Input: part model. Units: mm. Frame: model coordinates. Round coordinates to 2 decimals unless told otherwise and drop trailing zeros. Write each loop counter-clockwise with the first axis right and the second up, starting at its lowest first coordinate (ties: lowest second). Pieces come first, ordered by that corner, then holes. Notation, with made-up numbers: (16.5, -14) -> (67.5, -14) arc R10 cw to (67.5, -9) -> close; hole circle Ø9 at (27, 27). An arc over 180 degrees is marked (long way). Write item = value, one per line. Start each with the question number.
```python
from build123d import *

# Parameters (mm, degrees)
SKETCH1_R           = 2.265
BOSS_EXTRUDE1_DEPTH = 3
SKETCH2_W           = 6.5
SKETCH2_H           = 20
CUT_EXTRUDE1_DEPTH  = 3
BOSS_EXTRUDE2_DEPTH = 3
CUT_EXTRUDE2_DEPTH  = 3
SKETCH5_W           = 3
SKETCH5_H           = 20
BOSS_EXTRUDE3_DEPTH = 3
SKETCH6_W           = 27.010134686
SKETCH6_H           = 17.9
CUT_EXTRUDE3_DEPTH  = 3
SKETCH7_W           = 19.5
SKETCH7_H           = 14.6
CUT_EXTRUDE4_DEPTH  = 3
SKETCH8_W           = 19.5
SKETCH8_H           = 15.6
CUT_EXTRUDE5_DEPTH  = 3
SKETCH9_W           = 2.019620965
SKETCH9_H           = 0.574286347
CUT_EXTRUDE6_DEPTH  = 3
SKETCH10_W          = 15
SKETCH10_H          = 3
CUT_EXTRUDE7_DEPTH  = 3
FILLET1_R           = 0.6


with BuildPart() as part:
    # Sketch1 → Boss-Extrude1 (new body)
    with BuildSketch(Plane(origin=(0, 0, 0), x_dir=(1, 0, 0), z_dir=(0, 1, 0))):
        with BuildLine():
            Line((4.265, 0), (87.735, 0))
            ThreePointArc((87.735, 0), (95.015810422, 3.015810422), (92, -4.265))
            Line((92, -4.265), (92, -58.735))
            ThreePointArc((92, -58.735), (95.015810422, -66.015810422), (87.735, -63))
            Line((87.735, -63), (4.265, -63))
            ThreePointArc((4.265, -63), (-3.015810422, -66.015810422), (0, -58.735))
            Line((0, -58.735), (0, -4.265))
            ThreePointArc((0, -4.265), (-3.015810422, 3.015810422), (4.265, 0))
        make_face()
        with Locations(Location((0, 0, 0), (0, 0, 270))):
            Circle(SKETCH1_R, mode=Mode.SUBTRACT)
        with Locations(Location((92, 0, 0), (0, 0, 270))):
            Circle(SKETCH1_R, mode=Mode.SUBTRACT)
        with Locations(Location((92, -63, 0), (0, 0, 270))):
            Circle(SKETCH1_R, mode=Mode.SUBTRACT)
        with Locations(Location((0, -63, 0), (0, 0, 270))):
            Circle(SKETCH1_R, mode=Mode.SUBTRACT)
    extrude(amount=BOSS_EXTRUDE1_DEPTH)

    # Sketch2 → Cut-Extrude1 (cut)
    with BuildSketch(Plane(origin=(0, 3, 0), x_dir=(1, 0, 0), z_dir=(0, 1, 0))):
        with Locations((3.25, -31.5)):
            Rectangle(SKETCH2_W, SKETCH2_H)
    extrude(amount=-CUT_EXTRUDE1_DEPTH, mode=Mode.SUBTRACT)

    # Sketch3 → Boss-Extrude2 (add)
    with BuildSketch(Plane(origin=(0, 3, 0), x_dir=(1, 0, 0), z_dir=(0, 1, 0))):
        with BuildLine():
            Line((-2.7, -15.5), (0, -14.9))
            Line((0, -14.9), (0, -21.5))
            Line((0, -21.5), (-2.5, -21.5))
            ThreePointArc((-2.5, -21.5), (-2.853553391, -21.353553391), (-3, -21))
            Line((-3, -21), (-3, -15.8))
            ThreePointArc((-3, -15.8), (-2.912132034, -15.587867966), (-2.7, -15.5))
        make_face()
        with BuildLine():
            Line((-3, -42), (-3, -47.2))
            ThreePointArc((-3, -47.2), (-2.912132034, -47.412132034), (-2.7, -47.5))
            Line((-2.7, -47.5), (0, -48.1))
            Line((0, -48.1), (0, -41.5))
            Line((0, -41.5), (-2.5, -41.5))
            ThreePointArc((-2.5, -41.5), (-2.853553391, -41.646446609), (-3, -42))
        make_face()
    extrude(amount=-BOSS_EXTRUDE2_DEPTH)

    # Sketch4 → Cut-Extrude2 (cut)
    with BuildSketch(Plane(origin=(0, 3, 0), x_dir=(1, 0, 0), z_dir=(0, 1, 0))):
        with BuildLine():
            Line((6, -3), (64, -3))
            ThreePointArc((64, -3), (66.121320344, -3.878679656), (67, -6))
            Line((67, -6), (67, -57))
            ThreePointArc((67, -57), (66.121320344, -59.121320344), (64, -60))
            Line((64, -60), (6, -60))
            ThreePointArc((6, -60), (3.878679656, -59.121320344), (3, -57))
            Line((3, -57), (3, -6))
            ThreePointArc((3, -6), (3.878679656, -3.878679656), (6, -3))
        make_face()
    extrude(amount=-CUT_EXTRUDE2_DEPTH, mode=Mode.SUBTRACT)

    # Sketch5 → Boss-Extrude3 (add)
    with BuildSketch(Plane(origin=(0, 3, 0), x_dir=(1, 0, 0), z_dir=(0, 1, 0))):
        with Locations((1.5, -31.5)):
            Rectangle(SKETCH5_W, SKETCH5_H)
    extrude(amount=-BOSS_EXTRUDE3_DEPTH)

    # Sketch6 → Cut-Extrude3 (cut)
    with BuildSketch(Plane(origin=(0, 3, 0), x_dir=(1, 0, 0), z_dir=(0, 1, 0))):
        with Locations((82.505067343, -14.45)):
            Rectangle(SKETCH6_W, SKETCH6_H)
    extrude(amount=-CUT_EXTRUDE3_DEPTH, mode=Mode.SUBTRACT)

    # Sketch7 → Cut-Extrude4 (cut)
    with BuildSketch(Plane(origin=(0, 3, 0), x_dir=(1, 0, 0), z_dir=(0, 1, 0))):
        with Locations((82.25, -33.7)):
            Rectangle(SKETCH7_W, SKETCH7_H)
    extrude(amount=-CUT_EXTRUDE4_DEPTH, mode=Mode.SUBTRACT)

    # Sketch8 → Cut-Extrude5 (cut)
    with BuildSketch(Plane(origin=(0, 3, 0), x_dir=(1, 0, 0), z_dir=(0, 1, 0))):
        with Locations((82.25, -51.3)):
            Rectangle(SKETCH8_W, SKETCH8_H)
    extrude(amount=-CUT_EXTRUDE5_DEPTH, mode=Mode.SUBTRACT)

    # Sketch9 → Cut-Extrude6 (cut)
    with BuildSketch(Plane(origin=(0, 3, 0), x_dir=(1, 0, 0), z_dir=(0, 1, 0))):
        with Locations((93.009810483, -58.812856827)):
            Rectangle(SKETCH9_W, SKETCH9_H)
    extrude(amount=-CUT_EXTRUDE6_DEPTH, mode=Mode.SUBTRACT)

    # Sketch10 → Cut-Extrude7 (cut)
    with BuildSketch(Plane(origin=(0, 3, 0), x_dir=(1, 0, 0), z_dir=(0, 1, 0))):
        with Locations((53.5, -61.5)):
            Rectangle(SKETCH10_W, SKETCH10_H)
    extrude(amount=-CUT_EXTRUDE7_DEPTH, mode=Mode.SUBTRACT)

    # Fillet1
    fillet1_edges = [part.edges().sort_by_distance(p)[0] for p in [
        (0, 1.5, 41.5),
        (92, 1.5, 4.265),
        (0, 1.5, 21.5),
        (87.735, 1.5, 63),
        (4.265, 1.5, 63),
        (0, 1.5, 58.735),
        (0, 1.5, 4.265),
        (4.265, 1.5, 0),
        (87.735, 1.5, 0),
        (93.726332818, 1.5, 59.1),
        (0, 1.5, 14.9),
        (0, 1.5, 48.1),
    ]]
    fillet(fillet1_edges, radius=FILLET1_R)


solid = part.part
```
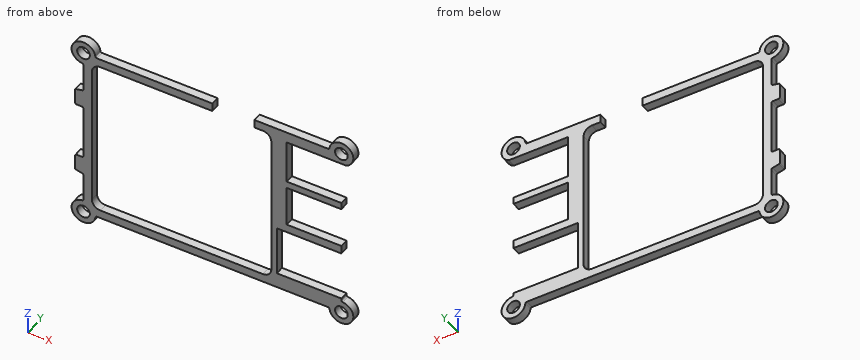
1. Line query: line 1 along Z through (x, y) = (77, 0.65); line 2 along X through (y, z) = (1.05, 24.5); line 3 along X through (y, z) = (1.75, 33). Output: solid intervals per line, ascending.
2. Section B-B (x = 43). Output: boundary loops of the cut face in (y, z).
3. Pin query (flat end, axial travel): P1, Ø0.9, axis at x = 84, y = 1.5, coming from the +Z side; P2, Ø1.5, axis at y = 2, z = 61, coming from the -X side; P3, Ø1.5, axis at y = 2, z = 10, coming from the +X side. Return the tip coordinate at first contact, or that it passes through.
4. Section C-C (y = 0.75). State how many separate pieces and enclosed holes the cut face has, then the cut area to 3 significant figures.
5. Section D-D (z = 62). Output: boundary loops of the cut face in (x, y), then the cut area to 3 significant figures.
6. Section A-A (z = 30). Output: boundary loops of the cut face in (x, y), then the cut area to 3 significant figures.
Check sheet entries:
q1.line_1 = 0 to 5.5, 23.4 to 26.4, 41 to 43.5, 59.1 to 63
q1.line_2 = 0 to 3, 67 to 92
q1.line_3 = 0 to 3, 67 to 72.5
q2.outline = (0, 0) -> (3, 0) -> (3, 3) -> (0, 3) -> close; (0, 60) -> (3, 60) -> (3, 63) -> (0, 63) -> close
q3.P1 = 63
q3.P2 = -4.08
q3.P3 = 69
q4.separate_pieces = 1
q4.enclosed_holes = 4
q4.area = 1,250 mm2
q5.outline = (-4.15, 0) -> (-2.03, 0) -> (-2.03, 3) -> (-4.15, 3) -> close; (2.03, 0) -> (46, 0) -> (46, 3) -> (2.03, 3) -> close; (61, 0) -> (89.97, 0) -> (89.97, 3) -> (61, 3) -> close; (94.03, 0) -> (96.15, 0) -> (96.15, 3) -> (94.03, 3) -> close
q5.area = 231 mm2
q6.outline = (0, 0) -> (3, 0) -> (3, 3) -> (0, 3) -> close; (67, 0) -> (72.5, 0) -> (72.5, 3) -> (67, 3) -> close
q6.area = 25.5 mm2
